For this review, take the finished solid that the model builds, in its own axes (mm). A direction names the side the tool comes from. Coordinates: 2 decimals unless noted, no trailing zeros. Write each loop counter-clockwise with the first axis right and the second up, starting at its lowest first coordinate (ties: lowest second). Pieces come first, ordered by that corner, then holes. Notation, with made-up numbers: (13.5, -23) -> (23.5, -23) arc R18 ccw to (23.5, -3) -> close; hole circle Ø7 at (62, 84.25). An arc over 180 degrees is marked (long way). Put each result on its own line as item: value. Start each with the question number.
Item 1: The part is to be moulded in two halves that separate along Y. For faces 3 (the flat face through (409.12, -42, 123)), 4 (the flat face through (4, -165.147, 123)), 5 (the flat face through (4, -38, 4)), say which applies: +Y half, -Y half, draft (parallel to the pull), parting line (faces both ways), or undercut.
Item 2: Consider section A-A on z = 180. Give the boundary of the cut face in (x, y), and give its area (3 significant figures).
Item 3: Consider section C-C on x = -151.5. Give the boundary of the cut face in (y, z).
Item 4: Consider section B-B on y = 24. Give the boundary of the cut face in (x, z).
Item 5: To check wall thickness, follow L1, parallel to X at y = 26, z = 236.5; L2, parallel to Y at x = 359.5, z = 188.5; L3, parallel to Z at x = 73.5, y = 16. State the ranges of each line that lie inside material, in increasing order.
Item 6: For faces 1 (the flat face through (4, 84.853, 123)), 2 (the flat face through (4, -163.147, 129)), list the 3-axis set-ups (+Z, -Z, +X, -X, +Y, -Y) from which the entire face can be reached by the end or side of a thin tool; tool diameter is ignored.
```python
from build123d import *

# Parameters (mm, degrees)
F0_W     = 800
F0_H     = 250
F1_DEPTH = 250
F2_W     = 796
F2_H     = 246
F3_DEPTH = 246
F4_W     = 10
F4_H     = 30
F5_DEPTH = 2


with BuildPart() as f1:
    # F0 (on Top) → F1 (new body)
    with BuildSketch(Plane.XY):
        with Locations((9.119717, -40.146783)):
            Rectangle(F0_W, F0_H)
    extrude(amount=F1_DEPTH)

    # F2 (on face) → F3 (cut)
    with BuildSketch(Plane.XY.offset(250)):
        with Locations((9.119717, -40.146783)):
            Rectangle(F2_W, F2_H)
    extrude(amount=-F3_DEPTH, mode=Mode.SUBTRACT)

    # F4 (on face) → F5 (cut, through all)
    with BuildSketch(Plane(origin=(0, 84.853217, 0), x_dir=(-1, 0, 0), z_dir=(0, 1, 0))):
        with Locations((-359.119717, 205)):
            Rectangle(F4_W, F4_H)
        with Locations((340.880283, 205)):
            Rectangle(F4_W, F4_H)
    extrude(amount=-F5_DEPTH, mode=Mode.SUBTRACT)


solid = f1.part
```
Return value:
1. face 3: draft
1. face 4: -Y half
1. face 5: undercut
2. outline: (-390.88, -165.15) -> (409.12, -165.15) -> (409.12, 84.85) -> (-390.88, 84.85) -> close; hole (-388.88, -163.15) -> (407.12, -163.15) -> (407.12, 82.85) -> (-388.88, 82.85) -> close
2. area: 4,180 mm^2
3. outline: (-165.15, 0) -> (84.85, 0) -> (84.85, 250) -> (82.85, 250) -> (82.85, 4) -> (-163.15, 4) -> (-163.15, 250) -> (-165.15, 250) -> close
4. outline: (-390.88, 0) -> (409.12, 0) -> (409.12, 250) -> (407.12, 250) -> (407.12, 4) -> (-388.88, 4) -> (-388.88, 250) -> (-390.88, 250) -> close
5. L1: -390.88 to -388.88, 407.12 to 409.12
5. L2: -165.15 to -163.15, 82.85 to 84.85
5. L3: 0 to 4
6. face 1: +Z, -Z, +X, -X, +Y
6. face 2: +Z
